```python
from build123d import *

# Parameters (mm, degrees)
SKETCH2_R           = 2.65
BOSS_EXTRUDE1_DEPTH = 2
BOSS_EXTRUDE2_DEPTH = 2
CHAMFER1_SIZE       = 4.5
CHAMFER1_SIZE2      = 0.956504528
BOSS_EXTRUDE3_DEPTH = 0.75


with BuildPart() as part:
    # Sketch2 → Boss-Extrude1 (new body)
    with BuildSketch(Plane(origin=(0, 0, 0), x_dir=(1, 0, 0), z_dir=(0, 1, 0))):
        with BuildLine():
            Line((-15.984695958, -228.591802117), (-17.334483725, -247.89466649))
            ThreePointArc((-17.334483725, -247.89466649), (0, -248.5), (17.334483725, -247.89466649))
            Line((17.334483725, -247.89466649), (15.984695958, -228.591802117))
            ThreePointArc((15.984695958, -228.591802117), (0, -229.15), (-15.984695958, -228.591802117))
        make_face()
        with Locations(Location((0, -236.25, 0), (0, 0, 270))):
            Circle(SKETCH2_R, mode=Mode.SUBTRACT)
    extrude(amount=BOSS_EXTRUDE1_DEPTH)

    # Sketch3 → Boss-Extrude2 (add)
    with BuildSketch(Plane(origin=(0, 0, 0), x_dir=(1, 0, 0), z_dir=(0, 1, 0))):
        with BuildLine():
            Line((-15.705670063, -224.601545916), (-15.984695958, -228.591802117))
            ThreePointArc((-15.984695958, -228.591802117), (0, -229.15), (15.984695958, -228.591802117))
            Line((15.984695958, -228.591802117), (15.705670063, -224.601545916))
            ThreePointArc((15.705670063, -224.601545916), (0, -225.15), (-15.705670063, -224.601545916))
        make_face()
    extrude(amount=BOSS_EXTRUDE2_DEPTH)

    # Chamfer1
    chamfer1_edges = [part.edges().sort_by_distance(p)[0] for p in [
        (0, 0, 225.15),
    ]]
    chamfer1_side = [part.faces().sort_by_distance(p)[0] for p in [
        (0, 0, 248.078921217),
    ]]
    chamfer(chamfer1_edges, length=CHAMFER1_SIZE, length2=CHAMFER1_SIZE2, reference=chamfer1_side[0])

    # Sketch4 → Boss-Extrude3 (add)
    with BuildSketch(Plane.XZ):
        with BuildLine():
            Line((-17.020664763, 243.406846238), (-16.985701357, 242.906846238))
            ThreePointArc((-16.985701357, 242.906846238), (0, 243.5), (16.985701357, 242.906846238))
            Line((16.985701357, 242.906846238), (17.020664763, 243.406846238))
            ThreePointArc((17.020664763, 243.406846238), (0, 244.001220949), (-17.020664763, 243.406846238))
        make_face()
    extrude(amount=BOSS_EXTRUDE3_DEPTH)


solid = part.part
```
The listing builds one solid part. Answer for the finished solid, in the listing's coordinates (mm). A direction names the side the tool comes from. Coordinates: 2 decimals unless noted, no trailing zeros. Loops run counter-clockwise (first coordinate to the right, second up) from the corner with the lowest first, then second, coordinate; pieces in that order, holes last. Notation, with made-up numbers: (67.5, 3.5) - (111.5, 3.5) arc R34 cw to (111.5, 34.5) - close; hole circle Ø7 at (-11.5, 22). An arc over 180 degrees is marked (long way). Write item = value, one per line.
1) Section A-A (x = 0) is taken. Determine the outline of the cut face in (y, z).
Responses:
outline = (-0.75, 243.5) - (0, 243.5) - (0, 238.9) - (2, 238.9) - (2, 248.5) - (0, 248.5) - (0, 244) - (-0.75, 244) - close; (0, 229.65) - (0.96, 225.15) - (2, 225.15) - (2, 233.6) - (0, 233.6) - close
2) Section B-B (y = 1.5) is taken. Determine the outline of the cut face in (x, z), plus the area to 3 significant figures.
Responses:
outline = (-17.33, 247.89) - (-15.71, 224.6) arc R225.15 cw to (15.71, 224.6) - (17.33, 247.89) arc R248.5 ccw to start; hole circle Ø5.3 at (0, 236.25)
area = 750 mm^2
3) Determine the mould class of faces 1 (the face through (0.1, 1, 233.6)), 2 (the face through (-0.2, 1, 248.5)), 3 (the face through (-0.2, -0.75, 243.7)) for opening direction X: pulls with the +X half, pulls with the -X half, needs draft (parallel to the pull), parting line crosses it, or undercut.
Responses:
face_1 = undercut
face_2 = parting line crosses it
face_3 = needs draft
4) Find the intervals of material crossed by line 1 along Y through (x, z) = (14, 242.5); line 2 along X through (y, z) = (0.85, 236.25); line 3 along Z through (x, y) = (-1.5, -0.25), in increasing order.
Responses:
line_1 = 0 to 2
line_2 = -16.52 to -2.65, 2.65 to 16.52
line_3 = 243.5 to 244
5) Section D-D (z = 230) is taken. Determine the outline of the cut face in (x, y).
Responses:
outline = (-16.08, 0) - (16.08, 0) - (16.08, 2) - (-16.08, 2) - close
6) Each of these flat-tipped pins is pushed along its axis until it touches: P1, Ø5.5, axis at x = 4.5, z = 245, coming from the -Y side; P2, Ø1, axis at x = -12.5, y = 1, coming from the -Z side; P3, Ø1, axis at x = 0.5, y = 1.5, coming from the -Z side. Where does it stop, or does it pass through?
Responses:
P1 = -0.75
P2 = 224.77
P3 = 225.15
7) Section C-C (z = 236.25) is taken. Determine the outline of the cut face in (x, y), plus the area to 3 significant figures.
Responses:
outline = (-16.52, 0) - (-2.65, 0) - (-2.65, 2) - (-16.52, 2) - close; (2.65, 0) - (16.52, 0) - (16.52, 2) - (2.65, 2) - close
area = 55.5 mm^2
8) Which of the six approach directions +Z, -Z, +X, -X, +Y, -Y give full straight-line access (tool end or side, diameter ignored) to faces 4 (the face through (0.222, 0.485, 227.368)), 5 (the face through (0.22, 1.47, 225.15))?
Responses:
face_4 = -Z, -Y
face_5 = -Z, +Y, -Y
